from build123d import *

# Parameters (mm, degrees)
SKETCH1_R               = 13.5
SKETCH1_R_2             = 1.25
BOSS_EXTRUDE2_DEPTH     = 2
SKETCH2_R               = 7.5
BOSS_EXTRUDE3_DEPTH     = 8.5
SKETCH4_R               = 2.5
CUT_EXTRUDE1_DEPTH      = 7.5
BOSS_EXTRUDE6_DEPTH     = 7.5
CUT_EXTRUDE2_DEPTH      = 7.5
CUT_EXTRUDE2_DEPTH_BACK = 11.75
SKETCH5_R               = 1
BOSS_EXTRUDE5_START     = 1.9
SKETCH7_R               = 13.5
SKETCH7_R_2             = 5.25
BOSS_EXTRUDE5_DEPTH     = 1.9
CUT_EXTRUDE3_DEPTH      = 8
FILLET1_R               = 2.5
SKETCH12_R              = 0.00537481
SKETCH12_R_2            = 0.008144056
SKETCH12_R_3            = 1.25
SKETCH12_R_4            = 0.012822725
CUT_EXTRUDE4_DEPTH      = 10
CIRPATTERN1_COUNT       = 4
SKETCH13_W              = 5.5
SKETCH13_H              = 2.4
SKETCH13_W_2            = 4.5
SKETCH13_H_2            = 2
CUT_EXTRUDE5_DEPTH      = 4
CUT_EXTRUDE6_DEPTH      = 2.4
CUT_EXTRUDE7_DEPTH      = 2


with BuildPart() as part:
    # Sketch1 → Boss-Extrude2 (new body)
    with BuildSketch(Plane(origin=(0, 0, 0), x_dir=(1, 0, 0), z_dir=(0, 1, 0))):
        with Locations(Location((0, 0, 0), (0, 0, 270))):
            Circle(SKETCH1_R)
        with Locations(Location((11.25, 0, 0), (0, 0, 270))):
            Circle(SKETCH1_R_2, mode=Mode.SUBTRACT)
        with Locations(Location((0, -11.25, 0), (0, 0, 270))):
            Circle(SKETCH1_R_2, mode=Mode.SUBTRACT)
        with Locations(Location((-11.25, 0, 0), (0, 0, 270))):
            Circle(SKETCH1_R_2, mode=Mode.SUBTRACT)
        with Locations(Location((0, 11.25, 0), (0, 0, 270))):
            Circle(SKETCH1_R_2, mode=Mode.SUBTRACT)
    extrude(amount=BOSS_EXTRUDE2_DEPTH)

    # Sketch2 → Boss-Extrude3 (add)
    with BuildSketch(Plane(origin=(0, 2, 0), x_dir=(1, 0, 0), z_dir=(0, 1, 0))):
        with Locations(Location((0, 0, 0), (0, 0, 270))):
            Circle(SKETCH2_R)
    extrude(amount=BOSS_EXTRUDE3_DEPTH)

    # Sketch4 → Cut-Extrude1 (cut)
    with BuildSketch(Plane(origin=(0, 10.5, 0), x_dir=(1, 0, 0), z_dir=(0, 1, 0))):
        with Locations(Location((0, 0, 0), (0, 0, 270))):
            Circle(SKETCH4_R)
    extrude(amount=-CUT_EXTRUDE1_DEPTH, mode=Mode.SUBTRACT)

    # Sketch16 → Boss-Extrude6 (add)
    with BuildSketch(Plane(origin=(0, 10.5, 0), x_dir=(1, 0, 0), z_dir=(0, 1, 0))):
        with BuildLine():
            Line((-1.086066966, 2.251767871), (1.141386704, 2.224238385))
            ThreePointArc((1.141386704, 2.224238385), (0.030895574, 2.499809085), (-1.086066966, 2.251767871))
        make_face()
    extrude(amount=-BOSS_EXTRUDE6_DEPTH)

    # Sketch5 → Cut-Extrude2 (cut, two sides: drawn at the far end of the back side and taken through both)
    with BuildSketch(Plane.XY.offset(-CUT_EXTRUDE2_DEPTH_BACK)):
        with Locations(Location((0, 6.914506731, 0), (0, 0, 180))):
            Circle(SKETCH5_R)
    extrude(amount=CUT_EXTRUDE2_DEPTH + CUT_EXTRUDE2_DEPTH_BACK, mode=Mode.SUBTRACT)

    # Sketch7 → Boss-Extrude5 (add)
    with BuildSketch(Plane.XZ.offset(BOSS_EXTRUDE5_START)):
        with Locations(Location((0, 0, 0), (0, 0, 270))):
            Circle(SKETCH7_R)
        with Locations(Location((0, 0, 0), (0, 0, 90))):
            Circle(SKETCH7_R_2, mode=Mode.SUBTRACT)
    extrude(amount=-BOSS_EXTRUDE5_DEPTH)

    # Sketch9 → Cut-Extrude3 (cut)
    with BuildSketch(Plane(origin=(0, 10.5, 0), x_dir=(1, 0, 0), z_dir=(0, 1, 0))):
        Polygon((-2.414753661, -0.64727487), (-2.414753661, 0.64727487), (-3.984419716, 0), align=None)
    extrude(amount=-CUT_EXTRUDE3_DEPTH, mode=Mode.SUBTRACT)

    # Fillet1
    fillet1_edges = [part.edges().sort_by_distance(p)[0] for p in [
        (0, 2, -7.5),
    ]]
    fillet(fillet1_edges, radius=FILLET1_R - 0.0001)  # a hair under: the kernel refuses the full size

    # Sketch12 → Cut-Extrude4 (cut)
    with BuildSketch(Plane(origin=(0, 0, 0), x_dir=(1, 0, 0), z_dir=(0, 1, 0))):
        with Locations(Location((-0.239113034, -10.028559531, 0), (0, 0, 101.087404696))):
            Circle(SKETCH12_R)
        with Locations(Location((-1.014615915, 11.966073133, 0), (0, 0, 144.78716899))):
            Circle(SKETCH12_R_2)
        with Locations(Location((-11, 0, 0), (0, 0, 264.260829523))):
            Circle(SKETCH12_R_3)
        with Locations(Location((10.492985163, 0.978537759, 0), (0, 0, 127.726196418))):
            Circle(SKETCH12_R_4)
    cut_extrude4 = extrude(amount=-CUT_EXTRUDE4_DEPTH, mode=Mode.SUBTRACT)

    # CirPattern1: Cut-Extrude4 ×4 about axis
    cirpattern1_axis = Axis((0, 0, 0), (0, 1, 0))
    for i in range(1, CIRPATTERN1_COUNT):
        add(cut_extrude4.rotate(cirpattern1_axis, i * 360 / CIRPATTERN1_COUNT), mode=Mode.SUBTRACT)

    # Sketch13 → Cut-Extrude5 (cut)
    with BuildSketch(Plane(origin=(0, 10.5, 0), x_dir=(1, 0, 0), z_dir=(0, 1, 0))):
        with Locations((0, 5)):
            Rectangle(SKETCH13_W, SKETCH13_H)
        with Locations((0.141735204, -5)):
            Rectangle(SKETCH13_W_2, SKETCH13_H_2)
    extrude(amount=-CUT_EXTRUDE5_DEPTH, mode=Mode.SUBTRACT)

    # Sketch14 → Cut-Extrude6 (cut)
    with BuildSketch(Plane(origin=(0, 0, -3.8), x_dir=(-1, 0, 0), z_dir=(0, 0, -1))):
        Polygon((2.721817224, 8.550063007), (-0.055524673, 10.089447729), (-2.777341897, 8.453891453), (-2.721817224, 5.278950455), (0.055524673, 3.739565732), (2.777341897, 5.375122009), align=None)
    extrude(amount=CUT_EXTRUDE6_DEPTH, mode=Mode.SUBTRACT)

    # Sketch15 → Cut-Extrude7 (cut)
    with BuildSketch(Plane.XY.offset(4)):
        Polygon((2.25, 8.213544837), (0, 9.512582942), (-2.25, 8.213544837), (-2.25, 5.615468625), (0, 4.31643052), (2.25, 5.615468625), align=None)
    extrude(amount=CUT_EXTRUDE7_DEPTH, mode=Mode.SUBTRACT)


solid = part.part
Part model, mm, in its own coordinate system. A direction names the side the tool comes from. Give positions to 0.01 mm unless a question says otherwise; leave off trailing zeros. Write each question's results on one line, items separated by ' | '. Start each with the question number.
Q1. Pull direction Y, two halves, no side cores. Call faces 3 (the face through (-2.25, 7, 5)), 4 (the face through (-1.916, 6.802, -1.606)), 5 (the face through (0.22, 7.89, -3.02)), 6 (the face through (-3, 2.5, 0)): +Y half, -Y half, draft (parallel to the pull), parting line (faces both ways), or undercut.
Q2. Which spindle directions (+Z, -Z, +X, -X, +Y, -Y) get a long thin tool onto all of the face, cutting with end or side? Do faces 1 (the face through (-2.87, 7.46, 6.93)), 2 (the face through (0.392, -0.937, -12.187)). Say none if no direction does.
Q3. Pin check, flat tips, straight feed: P1, Ø3.5, axis at x = -0.5, y = 6, coming from the -Z side; P2, Ø1.8, axis at x = 0, y = 6.91, coming from the +Z side; P3, Ø5, axis at x = -4.5, y = -0.5, coming from the -Z side; P4, Ø3, axis at x = 11, z = 0, coming from the +Y side. Stop position of each tip, or through.
Q4. Band-saw the part on A-A on y = -0.5. Count the separate pieces of the cut face and the enclosed holes in it, plus the area to 3 significant figures.
Q5. Wall check: L1, parallel to X at y = -0.85, z = 0; L2, parallel to Z at x = 0, y = 1.45; L3, parallel to Y at x = 0, z = -6.45. Give the ranges that are in metal, low to high.
Results are:
1) face 3: undercut | face 4: draft | face 5: undercut | face 6: +Y half
2) face 1: +Y | face 2: -Y
3) P1: stops at z = -7.51 | P2: passes through | P3: stops at z = -13.35 | P4: stops at y = 2.05
4) separate pieces: 1 | enclosed holes: 9 | area: 466 mm²
5) L1: x = -13.5 to -12.25, -9.75 to -5.25, 5.25 to 9.75, 12.25 to 13.5 | L2: z = -13.5 to -12.5, -10 to 10, 12.5 to 13.5 | L3: y = -1.9 to 5.91, 7.91 to 10.5
